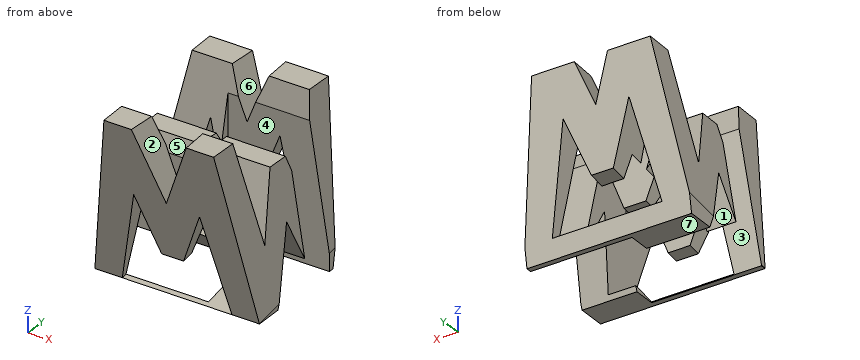
from build123d import *

# Parameters (mm, degrees)
F0_W     = 38.1
F0_H     = 38.1
F1_DEPTH = 38.1
F4_DEPTH = 38.1
F6_DEPTH = 38.1
F7_W     = 23.472134
F7_H     = 7.62
F7_W_2   = 25.4
F8_DEPTH = 38.1


with BuildPart() as f1:
    # F0 (on Front) → F1 (new body)
    with BuildSketch(Plane.XZ):
        with Locations((19.05, 19.05)):
            Rectangle(F0_W, F0_H)
    extrude(amount=F1_DEPTH)

    # F3 (on face) → F4 (cut)
    with BuildSketch(Plane.YZ.offset(38.1)):
        Polygon((-6.35, 38.1), (-31.75, 38.1), (-26.67, 14.267865), (-21.59, 28.575), (-16.51, 28.575), (-11.43, 14.267865), align=None)
        Polygon((-31.75, 0), (-38.1, 38.1), (-38.1, 0), align=None)
        Polygon((-19.05, 15.875), (-25.4, 0), (-12.7, 0), align=None)
        Polygon((0, 0), (0, 38.1), (-6.35, 0), align=None)
    extrude(amount=-F4_DEPTH, mode=Mode.SUBTRACT)

    # F5 (on face) → F6 (cut)
    with BuildSketch(Plane(origin=(0, -30.891892, -5.148649), x_dir=(1, 0, 0), z_dir=(0, -0.986394, -0.164399))):
        Polygon((11.43, 27.444668), (6.35, 5.219668), (31.75, 5.219668), (26.67, 27.444668), (21.59, 14.744668), (16.51, 14.744668), align=None)
        Polygon((25.4, 43.84521), (12.7, 43.84521), (19.05, 27.97021), align=None)
        Polygon((0, 43.84521), (0, 5.219668), (6.35, 43.84521), align=None)
        Polygon((31.75, 43.84521), (38.1, 5.219668), (38.1, 43.84521), align=None)
    extrude(amount=-F6_DEPTH, mode=Mode.SUBTRACT)

    # F7 (on offset) → F8 (cut)
    with BuildSketch(Plane.XY.offset(38.1)):
        with Locations((26.363933, -11.43)):
            Rectangle(F7_W, F7_H)
        with Locations((12.7, -26.67)):
            Rectangle(F7_W_2, F7_H)
    extrude(amount=-F8_DEPTH, mode=Mode.SUBTRACT)


solid = f1.part
Part model, mm, in its own coordinate system. Face numbers are marked on the shaded views. A direction names the side the tool comes from. Give positions to 0.01 mm unless a question says otherwise; leave off trailing zeros. Write each loop counter-clockwise with the first axis right and the second up, starting at its lowest first coordinate (ties: lowest second). Pieces come first, ordered by that corner, then holes.
1) Probe L1, parallel to Y at x = 19.5, z = 13; L2, parallel to Y at x = 4, z = 12; L3, parallel to Y at x = 27.5, z = 22.5. List the from-to ranges inside material, lowest first.
Resolved:
L1: y = -33.92 to -30.48, -22.86 to -20.2, -17.9 to -15.24
L2: y = -33.75 to -30.48, -22.86 to -20.6, -17.5 to -4.35
L3: y = -35.5 to -28.42, -23.75 to -15.24
2) Cut at A-A on y = -2.5. Write the cut outline in (x, z), then the cut area to 3 significant figures.
Resolved:
outline: (2.96, 23.1) - (10.46, 23.1) - (11.43, 27.41) - (13.13, 23.1) - (24.97, 23.1) - (26.67, 27.41) - (27.64, 23.1) - (35.14, 23.1) - (32.71, 38.1) - (23.06, 38.1) - (19.05, 27.94) - (15.04, 38.1) - (5.39, 38.1) - close
area: 394 mm2
3) Cut at C-C on y = -20. Write the cut outline in (x, z) (3 decimals), then the cut area to 3 significant figures.
Resolved:
outline: (1.872, 13.5) - (8.952, 13.5) - (11.43, 24.49) - (15.766, 13.5) - (22.334, 13.5) - (26.67, 24.49) - (29.148, 13.5) - (36.228, 13.5) - (33.784, 28.575) - (20.452, 28.575) - (19.05, 25.023) - (17.648, 28.575) - (4.316, 28.575) - close
area: 401 mm2
4) Pin check, flat tips, straight feed: pin 1 (20.5 mm diameter, centred on x = 14.5, z = 13, fed in from -Y) (3 decimals); pin 2 (1.5 mm diameter, centred on x = 30.5, y = -18, fed in from +Z) (3 decimals); pin 3 (2 mm diameter, centred on x = 18.5, z = 7.5, fed in from +Y); pin 4 (2 mm diameter, centred on y = -14, z = 21.5, fed in from +X). Stop position of each tip, or through.
Resolved:
pin 1: stops at y = -35.625
pin 2: stops at z = 28.575
pin 3: passes through
pin 4: stops at x = 14.63
5) Two-plate mould, pull along X, no slides. Class the marked faces 6 and 7: released by +X, released by -X, zero draft, split by the parting line, or undercut.
Resolved:
face 6: undercut
face 7: zero draft
6) Which spindle directions (+Z, -Z, +X, -X, +Y, -Y) get a long thin tool onto all of the face, cutting with end or side? Do the marked faces 1, 2, 3, 4 and 5. Say none if no direction does.
Resolved:
face 1: -Z, +X, -X
face 2: +Z, -Y
face 3: +Z, -Z, -X
face 4: +Z, -Z, +X
face 5: +Z, +X, -X
7) Cut at B-B on z = 13. State how many separate pieces and enclosed holes the cut face has, then the cut area to 3 significant figures.
Resolved:
separate pieces: 9
enclosed holes: 0
area: 338 mm2
